Read the model definition and answer for the solid it produces. Units are mm, in the model's axes. Face numbers are marked on the shaded views. A direction names the side the tool comes from. Coordinates: 2 decimals unless noted, no trailing zeros. Loops run counter-clockwise (first coordinate to the right, second up) from the corner with the lowest first, then second, coordinate; pieces in that order, holes last. Notation, with made-up numbers: (72.25, 6) -> (109.25, 6) arc R4 cw to (109.25, 12) -> close; hole circle Ø2 at (-14.75, -22.75). An arc over 180 degrees is marked (long way). One line per question, with ' | ' between items. Start each with the question number.
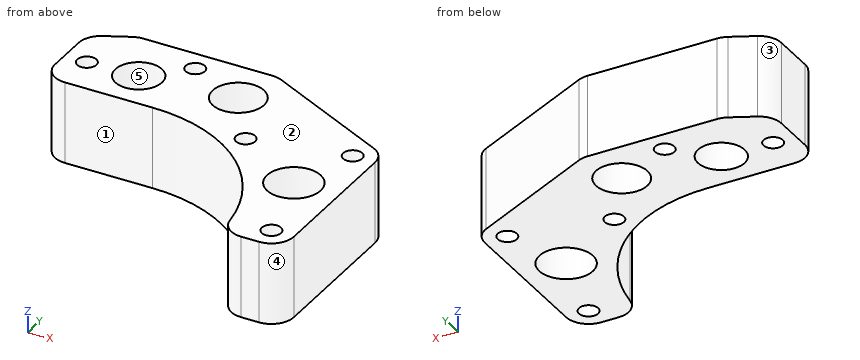
```python
from build123d import *

# Parameters (mm, degrees)
SKETCH_1_R           = 6
EXTRUDE_1_DEPTH      = 18.3
CUT_EXTRUDE_1_DEPTH  = 18.3
CUT_EXTRUDE_2_DEPTH  = 18.3
CUT_EXTRUDE_3_DEPTH  = 18.3
FILLET_1_R           = 2
CUT_EXTRUDE_4_DEPTH  = 18.3
CUT_EXTRUDE_5_DEPTH  = 18.3
CUT_EXTRUDE_6_DEPTH  = 60
CUT_EXTRUDE_8_DEPTH  = 104
SKETCH_10_R          = 2.15
CUT_EXTRUDE_9_DEPTH  = 144
FILLET_2_R           = 5
SKETCH_13_R          = 6
SKETCH_13_R_2        = 5.747449745
SKETCH_13_R_3        = 5.213004259
CUT_EXTRUDE_11_DEPTH = 70


with BuildPart() as part:
    # 草图1 → 凸台-拉伸1 (new body)
    with BuildSketch(Plane.XY):
        with BuildLine():
            Line((-56, 0), (-34.35, 0))
            ThreePointArc((-34.35, 0), (0, 34.35), (34.35, 0))
            Line((34.35, 0), (56, 0))
            Line((56, 0), (56, 56.65))
            Line((56, 56.65), (8.281928864, 111.239451243))
            ThreePointArc((8.281928864, 111.239451243), (0, 115), (-8.281928864, 111.239451243))
            Line((-8.281928864, 111.239451243), (-56, 56.65))
            Line((-56, 56.65), (-56, 0))
        make_face()
        with Locations((0, 104)):
            Circle(SKETCH_1_R, mode=Mode.SUBTRACT)
    extrude(amount=EXTRUDE_1_DEPTH)

    # 草图2 → 切除-拉伸1 (cut)
    with BuildSketch(Plane(origin=(0, 0, 0), x_dir=(-1, 0, 0), z_dir=(0, 0, -1))):
        with BuildLine():
            Line((56, 34.35), (0, 34.35))
            ThreePointArc((0, 34.35), (24.289117934, 24.289117934), (34.35, 0))
            Line((34.35, 0), (56, 0))
            Line((56, 0), (56, 34.35))
        make_face()
    extrude(amount=-CUT_EXTRUDE_1_DEPTH, mode=Mode.SUBTRACT)

    # 草图3 → 切除-拉伸2 (cut)
    with BuildSketch(Plane(origin=(0, 0, 0), x_dir=(-1, 0, 0), z_dir=(0, 0, -1))):
        Polygon((41, 34.35), (41, 59.35), (9.317845696, 109.846174099), (56, 56.65), (56, 34.35), align=None)
    extrude(amount=-CUT_EXTRUDE_2_DEPTH, mode=Mode.SUBTRACT)

    # 草图4 → 切除-拉伸3 (cut)
    with BuildSketch(Plane.XY.offset(18.3)):
        Polygon((-9.317845696, 109.846174099), (-8.855036315, 110.583816584), (-56, 56.65), align=None)
    extrude(amount=-CUT_EXTRUDE_3_DEPTH, mode=Mode.SUBTRACT)

    # 圆角1
    fillet_1_edges = [part.edges().sort_by_distance(p)[0] for p in [
        (-41, 34.35, 9.15),
    ]]
    fillet(fillet_1_edges, radius=FILLET_1_R)

    # 草图5 → 切除-拉伸4 (cut)
    with BuildSketch(Plane(origin=(0, 0, 0), x_dir=(-1, 0, 0), z_dir=(0, 0, -1))):
        Polygon((24.641777725, 34.35), (24.641777725, 85.422331825), (54.641777725, 59.35), (54.641777725, 34.35), align=None)
    extrude(amount=-CUT_EXTRUDE_4_DEPTH, mode=Mode.SUBTRACT)

    # 草图6 → 切除-拉伸5 (cut)
    with BuildSketch(Plane.XY.offset(18.3)):
        Polygon((-24.641777725, 56.346305337), (15.622574059, 56.346305337), (54.315270896, 37.471819075), (54.315270896, 119.471819075), (-24.641777725, 119.471819075), align=None)
    extrude(amount=-CUT_EXTRUDE_5_DEPTH, mode=Mode.SUBTRACT)

    # 草图7 → 切除-拉伸6 (cut)
    with BuildSketch(Plane.XY.offset(18.3)):
        Polygon((-15.622574059, 56.346305337), (-24.641777725, 51.946693793), (-24.641777725, 56.346305337), align=None)
    extrude(amount=-CUT_EXTRUDE_6_DEPTH, mode=Mode.SUBTRACT)

    # 草图9 → 切除-拉伸8 (cut)
    with BuildSketch(Plane.XY.offset(18.3)):
        Polygon((48, 0), (48, 40.552439024), (56, 36.65), (56, 0), align=None)
    extrude(amount=-CUT_EXTRUDE_8_DEPTH, mode=Mode.SUBTRACT)


with BuildPart() as cut_extrude_8_piece_1:
    # of the separate pieces the step leaves, piece 1, a body of its own (cut_extrude_8_pieces)
    add(part.part.solids().sort_by_distance((-24.641777725, 34.35, 0))[0])

    # 草图10 → 切除-拉伸9 (cut)
    with BuildSketch(Plane(origin=(0, 0, 0), x_dir=(-1, 0, 0), z_dir=(0, 0, -1))):
        with Locations((-43, 5)):
            Circle(SKETCH_10_R)
        with Locations((-43, 37.428295255)):
            Circle(SKETCH_10_R)
        with Locations((0, 51.346305337)):
            Circle(SKETCH_10_R)
        with Locations((19.641777725, 43.148346896)):
            Circle(SKETCH_10_R)
        with Locations((-21.597406613, 32.893381213)):
            Circle(SKETCH_10_R)
    extrude(amount=-CUT_EXTRUDE_9_DEPTH, mode=Mode.SUBTRACT)

    # 圆角2
    fillet_2_edges = [cut_extrude_8_piece_1.edges().sort_by_distance(p)[0] for p in [
        (48, 0, 9.15),
        (34.35, 0, 9.15),
        (-24.641777725, 34.35, 9.15),
        (48, 40.552439024, 9.15),
        (15.622574059, 56.346305337, 9.15),
        (-15.622574059, 56.346305337, 9.15),
        (-24.641777725, 51.946693793, 9.15),
    ]]
    fillet(fillet_2_edges, radius=FILLET_2_R)

    # 草图13 → 切除-拉伸11 (cut)
    with BuildSketch(Plane(origin=(0, 0, 0), x_dir=(-1, 0, 0), z_dir=(0, 0, -1))):
        with Locations((-38, 22.86749877)):
            Circle(SKETCH_13_R)
        with Locations((-12.747449745, 45.790830958)):
            Circle(SKETCH_13_R_2)
        with Locations((8.278773466, 43.563004259)):
            Circle(SKETCH_13_R_3)
    extrude(amount=-CUT_EXTRUDE_11_DEPTH, mode=Mode.SUBTRACT)


with BuildPart() as cut_extrude_8_piece_2:
    # of the separate pieces the step leaves, piece 2, a body of its own (cut_extrude_8_pieces)
    add(part.part.solids().sort_by_distance((54.315270896, 37.471819075, 0))[0])


solid = cut_extrude_8_piece_1.part
```
(1) Determine the mould class of the marked faces 3, 4 and 5 for opening direction X: +X half, -X half, draft (parallel to the pull), parting line (faces both ways), or undercut.
(2) Section B-B on z = 6 is taken. Give the number of separate pieces and of enclosed holes in the cut face, plus the area to 3 significant figures.
(3) Each of these flat-tipped pins is pushed along its axis until it touches: pin 1 Ø1 at (x, z) = (36, 2.5) entering from +Y; pin 2 Ø10 at (x, z) = (12, 6) entering from -Y; pin 3 Ø2 at (y, z) = (38, 12.5) entering from -X. Where does it stop, or does it pass through?
(4) Section A-A on x = 38 is taken. Write down the section's boundary in (y, z), plus the area to 3 significant figures.
(5) Find the intervals of material crossed by probe 1 along Y at (x, z) = (43.5, 15.25); probe 2 along X at (y, z) = (48, 8.25); probe 3 along X at (y, z) = (51, 8.25), in increasing order. Write a range as from..to.
(6) A tool of negligible diameter and unlimited length cuts with its end or side. For the marked faces 1 and 2, from which of +Z, -Z, +X, -X, +Y, -Y can it reach the whole face along a straight path? Write none if from no direction.
(7) Section C-C on x = 28 is taken. Write down the section's boundary in (y, z).
Working result:
1) face 3: -X half | face 4: +X half | face 5: undercut
2) separate pieces: 1 | enclosed holes: 8 | area: 1,650 mm2
3) pin 1: stops at y = 46.65 | pin 2: stops at y = 29.85 | pin 3: stops at x = -24.63
4) outline: (0.11, 0) -> (16.87, 0) -> (16.87, 18.3) -> (0.11, 18.3) -> close; (28.87, 0) -> (45.43, 0) -> (45.43, 18.3) -> (28.87, 18.3) -> close | area: 610 mm2
5) probe 1: y = 0.03..2.91, 7.09..20.47, 25.27..35.34, 39.52..42.75 | probe 2: x = -24.64..-11.02, -5.54..7.44, 18.05..32.73 | probe 3: x = -24.14..-2.12, 2.12..10.32, 15.18..26.58
6) face 1: +Z, -Z, -X, -Y | face 2: +Z, +X, -X, +Y, -Y
7) outline: (19.9, 0) -> (50.31, 0) -> (50.31, 18.3) -> (19.9, 18.3) -> close
